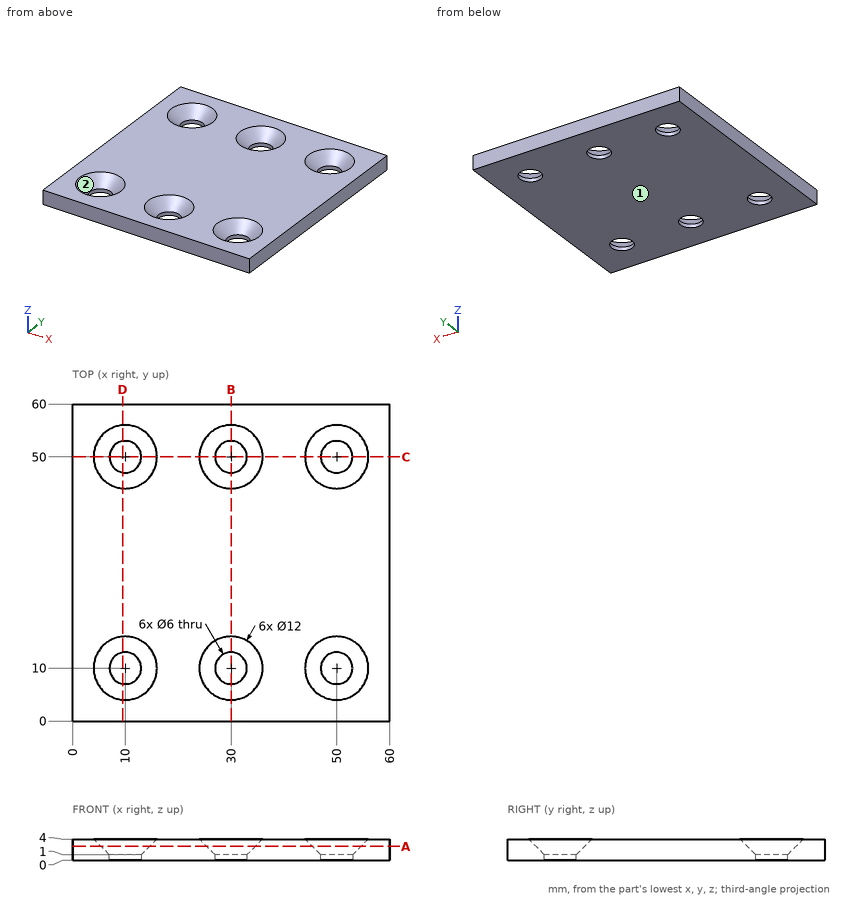
Source: three-view drawing plus pictorial views. Frame: mm from the lowest corner of the part. Round coordinates to 2 decimals unless told otherwise and drop trailing zeros. Order: outer loops, then holes, each group sorted by start corner. A loop starts at its lowest first (then second) coordinate and runs counter-clockwise, first axis right, second up. Notation, with made-up numbers: (10, -38) - (50, -38) arc R15 cw to (50, -16) - close; hole circle Ø2 at (54, 16). An arc over 180 degrees is marked (long way). Write each question's results on one line, items separated by ' | '.
Item 1: Section D-D, the plane x = 9.5. State how many separate pieces and enclosed holes the cut face has, and give its area (3 significant figures).
Completed:
separate pieces: 3 | enclosed holes: 0 | area: 175 mm^2
Item 2: First-contact query: pin 1 Ø8 at (x, y) = (50, 10) entering from +Z; pin 2 Ø9.5 at (x, y) = (50, 50) entering from +Z. Flat tips, straight axial feed; report the tip coordinate or a pass-through.
Completed:
pin 1: z = 2 | pin 2: z = 2.75
Item 3: Section A-A, the plane z = 2.6. Return the cut outline in (x, y), and give its area (3 significant figures).
Completed:
outline: (0, 0) - (60, 0) - (60, 60) - (0, 60) - close; hole circle Ø9.2 at (10, 10); hole circle Ø9.2 at (10, 50); hole circle Ø9.2 at (30, 10); hole circle Ø9.2 at (30, 50); hole circle Ø9.2 at (50, 10); hole circle Ø9.2 at (50, 50) | area: 3,200 mm^2
Item 4: Section C-C, the plane y = 50. Return the cut outline in (x, z).
Completed:
outline: (0, 0) - (7, 0) - (7, 1) - (4, 4) - (0, 4) - close; (13, 0) - (27, 0) - (27, 1) - (24, 4) - (16, 4) - (13, 1) - close; (33, 0) - (47, 0) - (47, 1) - (44, 4) - (36, 4) - (33, 1) - close; (53, 0) - (60, 0) - (60, 4) - (56, 4) - (53, 1) - close
Item 5: Material intervals for line 1 along Y through (x, z) = (30, 0.35); line 2 along X through (y, z) = (49, 1.05); line 3 along X through (y, z) = (11, 1.3), sorted ascending. Write a range as [from, to].
Completed:
line 1: [0, 7], [13, 47], [53, 60] | line 2: [0, 7.12], [12.88, 27.12], [32.88, 47.12], [52.88, 60] | line 3: [0, 6.86], [13.14, 26.86], [33.14, 46.86], [53.14, 60]
Item 6: Section B-B, the plane x = 30. Return the cut outline in (y, z), and give its area (3 significant figures).
Completed:
outline: (0, 0) - (7, 0) - (7, 1) - (4, 4) - (0, 4) - close; (13, 0) - (47, 0) - (47, 1) - (44, 4) - (16, 4) - (13, 1) - close; (53, 0) - (60, 0) - (60, 4) - (56, 4) - (53, 1) - close | area: 174 mm^2
Item 7: Mould query, pull axis X, two halves, no side actions, for the marked faces 1 and 2. Classes: pulls with the +X half, pulls with the -X half, needs draft (parallel to the pull), parting line crosses it, or undercut.
Completed:
face 1: needs draft | face 2: undercut
